Here's the drawing with two shaded views (mm, measured from the low corner). I have some questions. Give positions to 0.01 mm unless a question says otherwise; leave off trailing zeros. Write each loop counter-clockwise with the first axis right and the second up, starting at its lowest first coordinate (ties: lowest second). Pieces come first, ordered by that corner, then holes. Notation, with made-up numbers: (-38.75, 85.5) -> (17.25, 85.5) arc R15 cw to (17.25, 100.5) -> close; hole circle Ø10 at (-4.5, 81.5). An arc over 180 degrees is marked (long way). Put each result on its own line as item: value. Start each with the question number.
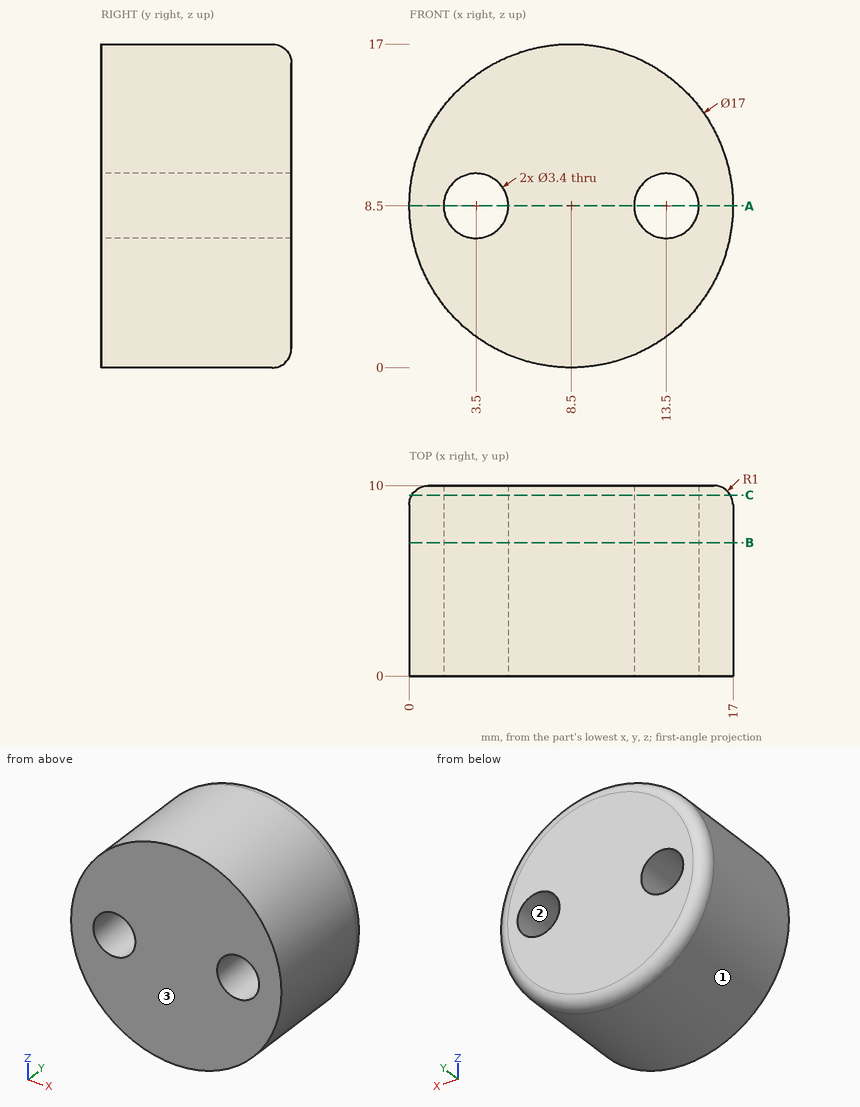
1) I want a section at C-C, the plane y = 9.5. Write out the boundary of the cut face in (x, z), and give its area (3 significant figures).
2) I need wall thicknesses on probe 1 along X at (y, z) = (1.75, 8.5); probe 2 along Z at (x, y) = (13.5, 2.75); probe 3 along X at (y, z) = (6.5, 9.5). Which ranges of each line are inside material? Lowest first, please.
3) I want a section at A-A, the plane z = 8.5. Write out the boundary of the cut face in (x, y), and give its area (3 significant figures).
4) I want a section at B-B, the plane y = 7. Write out the boundary of the cut face in (x, z), and give its area (3 significant figures).
5) Thinking about a two-plate mould opening in Z: for the marked faces 1, 2 and 3, which applies, released by +Z, released by -Z, zero draft, split by the parting line, or undercut?
6) I'm going to push flat-ended pins straight in: pin 1 Ø5.5 at (x, z) = (3.5, 8.5) entering from +Y; pin 2 Ø4 at (x, y) = (2.5, 4.5) entering from -Z; pin 3 Ø1.5 at (x, y) = (3.5, 6) entering from +Z; pin 4 Ø5 at (x, y) = (13, 3.5) entering from -Z. Where does each tip first touch, or does it pass through?
Established:
1. outline: circle Ø16.73 at (8.5, 8.5); hole circle Ø3.4 at (3.5, 8.5); hole circle Ø3.4 at (13.5, 8.5)
1. area: 202 mm2
2. probe 1: x = 0 to 1.8, 5.2 to 11.8, 15.2 to 17
2. probe 2: z = 1.63 to 6.8, 10.2 to 15.37
2. probe 3: x = 0.06 to 2.13, 4.87 to 12.13, 14.87 to 16.94
3. outline: (0, 0) -> (1.8, 0) -> (1.8, 10) -> (1, 10) arc R1 ccw to (0, 9) -> close; (5.2, 0) -> (11.8, 0) -> (11.8, 10) -> (5.2, 10) -> close; (15.2, 0) -> (17, 0) -> (17, 9) arc R1 ccw to (16, 10) -> (15.2, 10) -> close
3. area: 102 mm2
4. outline: circle Ø17 at (8.5, 8.5); hole circle Ø3.4 at (3.5, 8.5); hole circle Ø3.4 at (13.5, 8.5)
4. area: 209 mm2
5. face 1: split by the parting line
5. face 2: undercut
5. face 3: zero draft
6. pin 1: stops at y = 10
6. pin 2: stops at z = 1
6. pin 3: stops at z = 15.86
6. pin 4: stops at z = 0.24
